Source: CAD feature listing. Evaluate the final solid. Frame: model axes, mm. A direction names the side the tool comes from. Give positions to 0.01 mm unless a question says otherwise; leave off trailing zeros. Write each loop counter-clockwise with the first axis right and the second up, starting at its lowest first coordinate (ties: lowest second). Pieces come first, ordered by that corner, then holes. Notation, with made-up numbers: (67, 40) -> (95, 40) arc R21 ccw to (95, 65) -> close; hole circle Ø7 at (40.5, 4). An arc over 180 degrees is marked (long way). Answer as a JSON object with one key per item and string values. Group by question number.
Item 1: First-contact query: pin 1 Ø10 at (y, z) = (-3, 35) entering from -X; pin 2 Ø24 at (x, y) = (-10.5, -12) entering from +Z. Flat tips, straight axial feed; report the tip coordinate or a pass-through.
Item 2: Section query D-D on z = 31.5. Return the cut outline in (x, y), plus the area to 3 significant figures.
Item 3: Section query A-A on x = 0. Return the cut outline in (y, z), plus the area to 3 significant figures.
Item 4: Section query C-C on y = -34. Return the cut outline in (x, z).
Item 5: Ray query, probe 1 along Y at (x, z) = (0, 25); probe 2 along Z at (x, y) = (-13.5, -26); probe 3 along X at (y, z) = (6, 23.5). Return the intervals inside material, ascending. Write a range as from..to.
Item 6: Pull-direction query (Y, two-part tool) for faces 1 (the face through (10, 40, 22)), 2 (the face through (10, -40, 17)), 3 (the face through (10.752, 18.603, 16.803)), 4 (the face through (50, -1, 22)); classes: pulls with the +Y half, pulls with the -Y half, needs draft (parallel to the pull), parting line crosses it, or undercut.
Item 7: Access query for faces 5 (the face through (22.396, -26.174, 34.14)), 6 (the face through (32, 9, 44)). Directions: +Z, -Z, +X, -X, +Y, -Y. A direction counts if a zero-diameter tool reaches every point of the face in a straight line with its end or side. Return the directions, or none.
Item 8: Section query B-B on y = -3. Return the cut outline in (x, z).
from build123d import *

# Parameters (mm, degrees)
F0_W     = 100
F0_H     = 80
F0_R     = 20
F1_DEPTH = 44
F2_DEPTH = 44
F4_DEPTH = 20


with BuildPart() as f1:
    # F0 (on Top) → F1 (new body)
    with BuildSketch(Plane.XY):
        Rectangle(F0_W, F0_H)
        with Locations((0, 1.739223)):
            Circle(F0_R, mode=Mode.SUBTRACT)
    extrude(amount=F1_DEPTH)

    # F0 (on Top) → F2 (join)
    with BuildSketch(Plane.XY):
        Rectangle(F0_W, F0_H)
        with Locations((0, 1.739223)):
            Circle(F0_R, mode=Mode.SUBTRACT)
    extrude(amount=F2_DEPTH)

    # F3 (on face) → F4 (cut)
    with BuildSketch(Plane.XY.offset(44)):
        with BuildLine():
            Line((-3.760391, 21.382529), (-14, 40))
            Line((-14, 40), (-50, 40))
            Line((-50, 40), (-50, -40))
            Line((-50, -40), (30, -40))
            Line((30, -40), (14.575634, -11.955699))
            ThreePointArc((14.575634, -11.955699), (-17.524318, -7.899152), (-3.760391, 21.382529))
        make_face()
    extrude(amount=-F4_DEPTH, mode=Mode.SUBTRACT)


solid = f1.part
Worked answers:
{
 "1": {"pin 1": "x = 17.47", "pin 2": "z = 24"},
 "2": {"outline": "(-14, 40) -> (-3.76, 21.38) arc R20 cw to (14.58, -11.96) -> (30, -40) -> (50, -40) -> (50, 40) -> close", "area": "2,970 mm^2"},
 "3": {"outline": "(-40, 0) -> (-18.26, 0) -> (-18.26, 24) -> (-40, 24) -> close; (21.74, 0) -> (40, 0) -> (40, 44) -> (21.74, 44) -> close", "area": "1,330 mm^2"},
 "4": {"outline": "(-50, 0) -> (50, 0) -> (50, 44) -> (26.7, 44) -> (26.7, 24) -> (-50, 24) -> close"},
 "5": {"probe 1": "21.74..40", "probe 2": "0..24", "probe 3": "-50..-19.54, 19.54..50"},
 "6": {"face 1": "pulls with the +Y half", "face 2": "pulls with the -Y half", "face 3": "undercut", "face 4": "needs draft"},
 "7": {"face 5": "+Z, -X, -Y", "face 6": "+Z, +X, -X, +Y, -Y"},
 "8": {"outline": "(-50, 0) -> (-19.43, 0) -> (-19.43, 24) -> (-50, 24) -> close; (19.43, 0) -> (50, 0) -> (50, 44) -> (19.43, 44) -> close"}
}
